from build123d import *

# Parameters (mm, degrees)
SKETCH1_W           = 6.35
SKETCH1_H           = 25.4
BOSS_EXTRUDE1_DEPTH = 25.4
SKETCH4_R           = 6.441586538
CUT_EXTRUDE1_DEPTH  = 6.35
CUT_EXTRUDE2_REACH  = 8.35
SKETCH3_R           = 8.70585


with BuildPart() as part:
    # Sketch1 → Boss-Extrude1 (new body)
    with BuildSketch(Plane.XY):
        with Locations((8.322674216, -16.049389649)):
            Rectangle(SKETCH1_W, SKETCH1_H)
    extrude(amount=BOSS_EXTRUDE1_DEPTH)

    # Sketch4 → Cut-Extrude1 (cut)
    with BuildSketch(Plane.ZY.offset(-5.147674216)):
        with Locations((12.7, -16.049389649)):
            Circle(SKETCH4_R)
    extrude(amount=-CUT_EXTRUDE1_DEPTH, mode=Mode.SUBTRACT)

    # Sketch3 → Cut-Extrude2 (cut, up to next)
    with BuildSketch(Plane.ZY.offset(-5.147674216), mode=Mode.PRIVATE) as cut_extrude2_sk1:
        with Locations((12.7, -16.049389649)):
            Circle(SKETCH3_R)
    cut_extrude2_tool1 = extrude(cut_extrude2_sk1.sketch, amount=-CUT_EXTRUDE2_REACH, mode=Mode.PRIVATE) & part.part
    add(cut_extrude2_tool1.solids().sort_by_distance((5.147674, -16.04939, 12.7))[0], mode=Mode.SUBTRACT)


solid = part.part
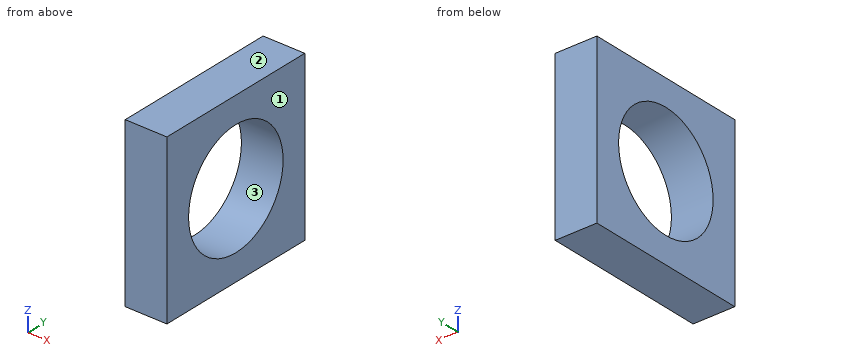
Build history of the part. All positions in model axes, mm. Face numbers are marked on the shaded views. Give positions to 0.01 mm unless a question says otherwise; leave off trailing zeros. Loops run counter-clockwise (first coordinate to the right, second up) from the corner with the lowest first, then second, coordinate; pieces in that order, holes last. Notation, with made-up numbers: (77.25, 81) -> (116.25, 81) arc R17 ccw to (116.25, 97) -> close; hole circle Ø1 at (15.5, 51.25). An arc over 180 degrees is marked (long way). Answer in a Markdown table with one row per item.
Item 1: Slice it at A-A on z = 12.7. Write the cut outline in (x, y), plus the area to 3 significant figures.
Findings below:
| item | result |
|---|---|
| outline | (5.15, -28.75) -> (11.5, -28.75) -> (11.5, -24.76) -> (5.15, -24.76) -> close; (5.15, -7.34) -> (11.5, -7.34) -> (11.5, -3.35) -> (5.15, -3.35) -> close |
| area | 50.7 mm² |
Item 2: Slice it at B-B on y = -9. Write the cut outline in (x, z), plus the area to 3 significant figures.
Findings below:
| item | result |
|---|---|
| outline | (5.15, 0) -> (11.5, 0) -> (11.5, 7.59) -> (5.15, 7.59) -> close; (5.15, 17.81) -> (11.5, 17.81) -> (11.5, 25.4) -> (5.15, 25.4) -> close |
| area | 96.4 mm² |
Item 3: Probe line 1 along Y through (x, z) = (6.75, 12.7); line 2 along Z through (x, y) = (6.75, -16); line 3 along Z through (x, y) = (8.75, -13.5). List the from-to ranges inside material, lowest first. Write a range as [from, to].
Findings below:
| item | result |
|---|---|
| line 1 | y = [-28.75, -24.76], [-7.34, -3.35] |
| line 2 | z = [0, 3.99], [21.41, 25.4] |
| line 3 | z = [0, 4.38], [21.02, 25.4] |
Item 4: Mould opens along Z. For the marked faces 1, 2 and 3 say: pulls with the +Z half, pulls with the -Z half, needs draft (parallel to the pull), parting line crosses it, or undercut.
Findings below:
| item | result |
|---|---|
| face 1 | needs draft |
| face 2 | pulls with the +Z half |
| face 3 | undercut |
Item 5: Slice it at C-C on x = 7.75. Write the cut outline in (y, z), plus the area to 3 significant figures.
Findings below:
| item | result |
|---|---|
| outline | (-28.75, 0) -> (-3.35, 0) -> (-3.35, 25.4) -> (-28.75, 25.4) -> close; hole circle Ø17.41 at (-16.05, 12.7) |
| area | 407 mm² |
